from build123d import *
from build123d import SkipClean  # not in build123d's __all__

# Parameters (mm, degrees)
F0_R     = 88.295
F1_DEPTH = 60
F2_R     = 2.5
F3_DEPTH = 300
F4_DEPTH = 300
F6_DEPTH = 300
F7_DEPTH = 300


with BuildPart() as f1:
    # F0 (on Front) → F1 (new body)
    with BuildSketch(Plane.XZ):
        Circle(F0_R)
        with BuildLine():
            ThreePointArc((80, 30.9964840748), (84.3338070557, 15.7667692474), (85.795, 0))
            ThreePointArc((85.795, 0), (-84.3338070557, -15.7667692474), (80, 30.9964840748))
        make_face(mode=Mode.SUBTRACT)
    extrude(amount=F1_DEPTH)

    # F2 (on Right) → F3 (cut)
    with BuildSketch(Plane.YZ):
        with Locations((-55, 0)):
            Circle(F2_R)
    extrude(amount=-F3_DEPTH, mode=Mode.SUBTRACT)

    # F2 (on Right) → F4 (cut)
    with BuildSketch(Plane.YZ):
        with Locations((-55, 0)):
            Circle(F2_R)
    with SkipClean():  # cleaning this boolean's faces spoils the solid; the shape is the same uncleaned
        extrude(amount=F4_DEPTH, mode=Mode.SUBTRACT)

    # F5 (on Top) → F6 (cut)
    with BuildSketch(Plane.XY):
        with BuildLine():
            ThreePointArc((0, -52.5), (-1.767766953, -56.767766953), (2.5, -55))
            ThreePointArc((2.5, -55), (1.767766953, -53.232233047), (0, -52.5))
        make_face()
    with SkipClean():  # cleaning this boolean's faces spoils the solid; the shape is the same uncleaned
        extrude(amount=-F6_DEPTH, mode=Mode.SUBTRACT)

    # F5 (on Top) → F7 (cut)
    with BuildSketch(Plane.XY):
        with BuildLine():
            ThreePointArc((0, -52.5), (-1.767766953, -56.767766953), (2.5, -55))
            ThreePointArc((2.5, -55), (1.767766953, -53.232233047), (0, -52.5))
        make_face()
    with SkipClean():  # cleaning this boolean's faces spoils the solid; the shape is the same uncleaned
        extrude(amount=F7_DEPTH, mode=Mode.SUBTRACT)


solid = f1.part
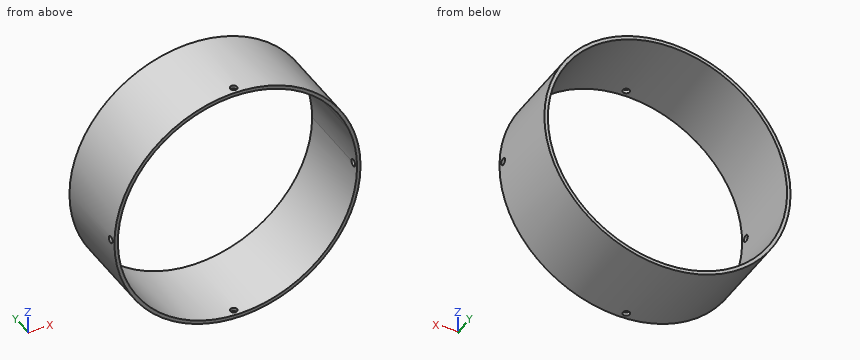
Build history of the part. All positions in model axes, mm. Give positions to 0.01 mm unless a question says otherwise; leave off trailing zeros. Loops run counter-clockwise (first coordinate to the right, second up) from the corner with the lowest first, then second, coordinate; pieces in that order, holes last. Notation, with made-up numbers: (68.5, -18) -> (96.5, -18) arc R12 cw to (96.5, -5) -> close; hole circle Ø3 at (69.25, 18). An arc over 180 degrees is marked (long way). Answer in a Markdown table with one row per item.
Item 1: Flat gauge pins, fed straight in: P1, Ø12, axis at x = -43, y = -13.5, coming from the +Z side; P2, Ø1.5, axis at x = 53, y = -18, coming from the -Z side; P3, Ø12, axis at x = -18, y = -51.5, coming from the -Z side; P4, Ø4.5, axis at y = -55, z = 0, coming from the -X side. Where does each tip first touch, or does it go through?
Findings below:
| item | result |
|---|---|
| P1 | stops at z = 80.17 |
| P2 | stops at z = -71.18 |
| P3 | stops at z = -87.48 |
| P4 | passes through |
Item 2: Slice it at B-B on x = 65.5. Write the cut outline in (y, z).
Findings below:
| item | result |
|---|---|
| outline | (-60, -59.21) -> (0, -59.21) -> (0, -55.41) -> (-60, -55.41) -> close; (-60, 55.41) -> (0, 55.41) -> (0, 59.21) -> (-60, 59.21) -> close |
Item 3: Probe line 1 along Y through (x, z) = (0, -87); line 2 along Z through (x, y) = (0, -17.5) (3 decimals); line 3 along Z through (x, y) = (-54, -56). List the from-to ranges inside material, lowest first. Write a range as [from, to].
Findings below:
| item | result |
|---|---|
| line 1 | y = [-60, -57.5], [-52.5, 0] |
| line 2 | z = [-88.295, -85.795], [85.795, 88.295] |
| line 3 | z = [-69.86, -66.67], [66.67, 69.86] |
Item 4: Slice it at A-A on z = 39. Write the cut outline in (x, y).
Findings below:
| item | result |
|---|---|
| outline | (-79.21, -60) -> (-76.42, -60) -> (-76.42, 0) -> (-79.21, 0) -> close; (76.42, -60) -> (79.21, -60) -> (79.21, 0) -> (76.42, 0) -> close |
Item 5: Slice it at C-C on y = -33. Write the cut outline in (x, z) (3 decimals).
Findings below:
| item | result |
|---|---|
| outline | circle Ø176.59 at (0, 0); hole circle Ø171.59 at (0, 0) |
